from build123d import *

# Parameters (mm, degrees)
IZIM1_W                     = 51
IZIM1_H                     = 51
Y_KSEKLIK_EKSTR_ZYON1_DEPTH = 51
IZIM2_W                     = 54.245036078
IZIM2_H                     = 53.426157313
KES_EKSTR_ZYON1_DEPTH       = 51
IZIM3_R                     = 11
IZIM3_R_2                   = 2
KES_EKSTR_ZYON2_DEPTH       = 51
PAH1_SIZE                   = 5
PAH2_SIZE                   = 5
KES_EKSTR_ZYON3_DEPTH       = 51


with BuildPart() as part:
    # Çizim1 → Yükseklik-Ekstrüzyon1 (new body)
    with BuildSketch(Plane.XY):
        Rectangle(IZIM1_W, IZIM1_H)
    extrude(amount=Y_KSEKLIK_EKSTR_ZYON1_DEPTH)

    # Çizim2 → Kes-Ekstrüzyon1 (cut)
    with BuildSketch(Plane.ZY.offset(25.5)):
        with Locations((20.877481961, 4.213078657)):
            Rectangle(IZIM2_W, IZIM2_H)
    extrude(amount=-KES_EKSTR_ZYON1_DEPTH, mode=Mode.SUBTRACT)

    # Çizim3 → Kes-Ekstrüzyon2 (cut)
    with BuildSketch(Plane.XY.offset(51)):
        with Locations((0, 4.5)):
            Circle(IZIM3_R)
        with Locations((-15.5, 20)):
            Circle(IZIM3_R_2)
        with Locations((15.5, 20)):
            Circle(IZIM3_R_2)
        with Locations((-15.5, -11)):
            Circle(IZIM3_R_2)
        with Locations((15.5, -11)):
            Circle(IZIM3_R_2)
    extrude(amount=-KES_EKSTR_ZYON2_DEPTH, mode=Mode.SUBTRACT)

    # Pah1
    pah1_edges = [part.edges().sort_by_distance(p)[0] for p in [
        (-25.5, 25.5, 49.5),
    ]]
    chamfer(pah1_edges, length=PAH1_SIZE)

    # Pah2
    pah2_edges = [part.edges().sort_by_distance(p)[0] for p in [
        (-25.5, -24, 0),
        (25.5, -24, 0),
        (25.5, 25.5, 49.5),
    ]]
    chamfer(pah2_edges, length=PAH2_SIZE)

    # Çizim4 → Kes-Ekstrüzyon3 (cut)
    with BuildSketch(Plane.XZ.offset(25.5)):
        with BuildLine():
            Line((-12.865, 39), (-12.865, 9))
            ThreePointArc((-12.865, 9), (-15.015, 6.85), (-17.165, 9))
            Line((-17.165, 9), (-17.165, 39))
            ThreePointArc((-17.165, 39), (-15.015, 41.15), (-12.865, 39))
        make_face()
        with BuildLine():
            Line((12.865, 39), (12.865, 9))
            ThreePointArc((12.865, 9), (15.015, 6.85), (17.165, 9))
            Line((17.165, 9), (17.165, 39))
            ThreePointArc((17.165, 39), (15.015, 41.15), (12.865, 39))
        make_face()
    extrude(amount=-KES_EKSTR_ZYON3_DEPTH, mode=Mode.SUBTRACT)


solid = part.part
The listing builds one solid part. Answer for the finished solid, in the listing's coordinates (mm). A direction names the side the tool comes from. Coordinates: 2 decimals unless noted, no trailing zeros. Write each loop counter-clockwise with the first axis right and the second up, starting at its lowest first coordinate (ties: lowest second). Pieces come first, ordered by that corner, then holes. Notation, with made-up numbers: (-38, 63) - (-1, 63) arc R13 cw to (-1, 69) - close; hole circle Ø4 at (-28, -31.5). An arc over 180 degrees is marked (long way). Answer as CSV lines item,"result".
1. Find section A-A (y = -11). Give the vertices of the cut face in (x, z), plus the area to 3 significant figures.
Computed values:
outline,"(-25.5, 48) - (-17.5, 48) - (-17.5, 51) - (-25.5, 51) - close; (-13.5, 48) - (13.5, 48) - (13.5, 51) - (-13.5, 51) - close; (17.5, 48) - (25.5, 48) - (25.5, 51) - (17.5, 51) - close"
area,"129 mm²"
2. Find section D-D (x = 15.5). Give the vertices of the cut face in (y, z), plus the area to 3 significant figures.
Computed values:
outline,"(-25.5, 0) - (-22.5, 0) - (-22.5, 6.91) - (-25.5, 6.91) - close; (-25.5, 41.09) - (-22.5, 41.09) - (-22.5, 48) - (-13, 48) - (-13, 51) - (-25.5, 51) - close; (-9, 48) - (18, 48) - (18, 51) - (-9, 51) - close; (22, 48) - (25.5, 48) - (25.5, 51) - (22, 51) - close"
area,"170 mm²"
3. Determine the mould class of faces 4 (the cylindrical face through (-2.38, -6.24, 49.52)), 5 (the cylindrical face through (-15.76, 21.983, 49.521)), 6 (the flat face through (0, -10, 48)), 7 (the flat face through (25.5, -23, 38)) for opening direction X: +X half, -X half, draft (parallel to the pull), parting line (faces both ways), or undercut.
Computed values:
face 4,"undercut"
face 5,"undercut"
face 6,"draft"
face 7,"+X half"
4. A tool of negligible diameter and unlimited length cuts with its end or side. For faces 1 (the flat face through (0, -22.5, 24)), 2 (the flat face through (0, 25.5, 49)), 3 (the flat face through (-17.165, -24, 24)), from which of +Z, -Z, +X, -X, +Y, -Y can it reach the whole face along a straight path? Write none if from no direction.
Computed values:
face 1,"-Z, +X, -X, +Y"
face 2,"+Z, -Z, +X, -X, +Y"
face 3,"+Y, -Y"
5. Given P1, Ø12, axis at x = 7.5, z = 13, coming from the +Y side; P2, Ø3, axis at x = -17, y = -20, coming from the -Z side, each flat-ended and moving along its own axis, determine where each tip first touches the part or whether it passes through.
Computed values:
P1,"stops at y = -22.5"
P2,"stops at z = 48"
6. Find section C-C (x = 10). Give the vertices of the cut face in (y, z).
Computed values:
outline,"(-25.5, 0) - (-22.5, 0) - (-22.5, 48) - (-0.08, 48) - (-0.08, 51) - (-25.5, 51) - close; (9.08, 48) - (25.5, 48) - (25.5, 51) - (9.08, 51) - close"
7. Find section B-B (z = 19.5). Give the vertices of the cut face in (x, y) (3 decimals), plus the area to 3 significant figures.
Computed values:
outline,"(-25.5, -25.5) - (-17.165, -25.5) - (-17.165, -22.5) - (-25.5, -22.5) - close; (-12.865, -25.5) - (12.865, -25.5) - (12.865, -22.5) - (-12.865, -22.5) - close; (17.165, -25.5) - (25.5, -25.5) - (25.5, -22.5) - (17.165, -22.5) - close"
area,"127 mm²"
8. Straight lines are drawn through the part: line 1 (Y direction, x = -15.5, z = 49.8); line 2 (Y direction, x = -15, z = 49); line 3 (Y direction, x = 11.5, z = 12). For each, find the intervals that lie inside material, in ascending order. Write a range as [from, to].
Computed values:
line 1,"y = [-25.5, -13], [-9, 18], [22, 25.5]"
line 2,"y = [-25.5, -12.94], [-9.06, 18.06], [21.94, 25.5]"
line 3,"y = [-25.5, -22.5]"
